Part model, mm, in its own coordinate system. A direction names the side the tool comes from. Give positions to 0.01 mm unless a question says otherwise; leave off trailing zeros. Write each loop counter-clockwise with the first axis right and the second up, starting at its lowest first coordinate (ties: lowest second). Pieces come first, ordered by that corner, then holes. Notation, with made-up numbers: M -23,-9 L -6,-9 A11 cw -6,11 Z; hole C 6.25,-5.75 d4. An arc over 180 degrees is marked long. Answer as CSV lines item,"result". Start each with the question number.
Item 1: Two-plate mould, pull along Y, no slides. Class faces 4 (the cylindrical face through (8.652, 16.634, -7.472)), 5 (the flat face through (0, 3, 0)), 6 (the cylindrical face through (0.16, 13.74, -3.86)): +Y half, -Y half, draft (parallel to the pull), parting line (faces both ways), or undercut.
Item 2: Pin check, flat tips, straight feed: pin 1 (8 mm diameter, centred on x = 5, y = 8, fed in from +Z); pin 2 (10 mm diameter, centred on y = -14.5, z = -10, fed in from +X); pin 3 (2 mm diameter, centred on x = 6.5, z = -9, fed in from +Y); pin 4 (4 mm diameter, centred on x = 0, y = -12.5, fed in from -Z). Stop position of each tip, or through.
Item 3: Wall check: L1, parallel to Y at x = 0, z = -10.5; L2, parallel to X at y = -0.5, z = -6; L3, parallel to Z at x = 3.5, y = -17. Give the ranges that are in metal, low to high. Write a range as from..to.
Item 4: 3-axis set-ups, long thin cutter, end or side, ignore diameter. For faces 1 (the cylindrical face through (0.16, -11.26, -3.86)), 2 (the cylindrical face through (-14.274, -0.628, -9.938)), 3 (the cylindrical face through (5.723, -1.802, -42.708)): which of +Z, -Z, +X, -X, +Y, -Y reach the whole face in a straight line?
Item 5: Band-saw the part on A-A, the plane z = -17.5. List the corners of the cut face in (x, y).
from build123d import *

# Parameters (mm, degrees)
M3X0_5_TAPPED_HOLE1_D     = 2.5
M3X0_5_TAPPED_HOLE1_DEPTH = 7.62
M3X0_5_TAPPED_HOLE1_TIP   = 0.751075774
CUT_EXTRUDE1_REACH        = 54.879
SKETCH5_R                 = 2.49301


with BuildPart() as part:
    # Sketch1 → Revolve1 (revolve)
    with BuildSketch(Plane(origin=(0, 0, 0), x_dir=(0, 0, -1), z_dir=(1, 0, 0)), mode=Mode.PRIVATE) as revolve1_sk:
        Polygon((0, 15.574573519), (0, 0), (45.75, 0), (45.75, 2.49), (45.75, 6), (39.75, 6), (38.389, 18.75), (10.389, 18.75), (10.389, 14.2875), (9.5, 14.2875), (9.5, 18.75), (5.5, 18.75), align=None)
    revolve(revolve1_sk.sketch.rotate(Axis((0, 0, 0), (0, 0, -1)), 90), axis=Axis((0, 0, 0), (0, 0, -1)))

    # M3x0.5 Tapped Hole1
    with Locations(Plane.XY):
        with Locations((0, 12.5), (12.5, 0), (-12.5, 0), (0, -12.5)):
            Hole(M3X0_5_TAPPED_HOLE1_D / 2, depth=M3X0_5_TAPPED_HOLE1_DEPTH)
            with Locations((0, 0, -(M3X0_5_TAPPED_HOLE1_DEPTH + M3X0_5_TAPPED_HOLE1_TIP / 2))):  # 118° drill point
                Cone(0, M3X0_5_TAPPED_HOLE1_D / 2, M3X0_5_TAPPED_HOLE1_TIP, mode=Mode.SUBTRACT)

    # Sketch5 → Cut-Extrude1 (cut, up to next)
    with BuildSketch(Plane.XY, mode=Mode.PRIVATE) as cut_extrude1_sk1:
        Circle(SKETCH5_R)
    cut_extrude1_tool1 = extrude(cut_extrude1_sk1.sketch, amount=-CUT_EXTRUDE1_REACH, mode=Mode.PRIVATE) & part.part
    add(cut_extrude1_tool1.solids().sort_by_distance((0, 0, 0))[0], mode=Mode.SUBTRACT)


solid = part.part
Output:
1,face 4,"parting line"
1,face 5,"draft"
1,face 6,"undercut"
2,pin 1,"z = 0"
2,pin 2,"x = 16.16"
2,pin 3,"y = 17.93"
2,pin 4,"z = -39.27"
3,L1,"-18.75..-2.49, 2.49..18.75"
3,L2,"-18.74..-13.65, -11.35..-2.44, 2.44..11.35, 13.65..18.74"
3,L3,"-38.54..-10.39, -9.5..-3.09"
4,face 1,"+Z"
4,face 2,"none"
4,face 3,"-Z"
5,outline,"C 0,0 d37.5; hole C 0,0 d4.99"
